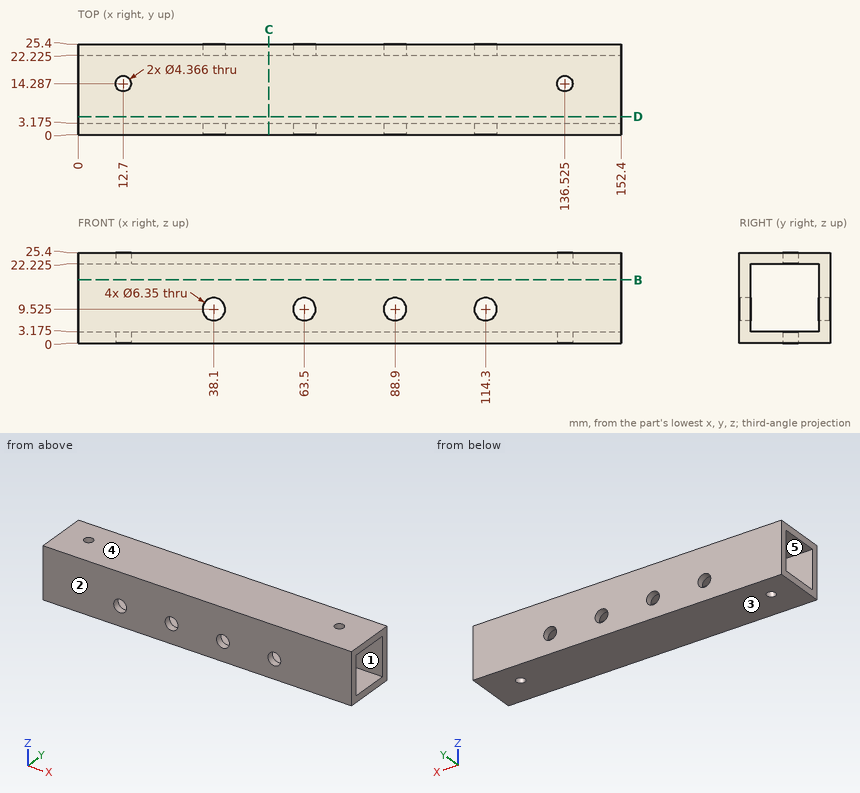
Can you work these out from the drawing? Everything is in mm from the part's minimum corner. A direction names the side the tool comes from. Round coordinates to 2 decimals unless told otherwise and drop trailing zeros. Loops run counter-clockwise (first coordinate to the right, second up) from the corner with the lowest first, then second, coordinate; pieces in that order, holes last. Notation, with made-up numbers: M 85.5,21.5 L 127.5,21.5 A26 cw 127.5,58.5 Z; hole C -11,-14 d1. An arc over 180 degrees is marked long. Answer in a Markdown table with one row per item.
1. If we section it at C-C, the plane x = 53.5: Please give me the cut outline in (y, z) (1 decimal).
Established:
| item | result |
|---|---|
| outline | M 0,0 L 25.4,0 L 25.4,25.4 L 0,25.4 Z; hole M 3.2,3.2 L 22.2,3.2 L 22.2,22.2 L 3.2,22.2 Z |
2. On a 3-axis mill with a long thin cutter (end or side, diameter ignored), from which of +Z, -Z, +X, -X, +Y, -Y can I reach the whole of each face in a straight line? I mean the marked faces 4 and 5. Say none if no direction works.
Established:
| item | result |
|---|---|
| face 4 | +Z, +X, -X, +Y, -Y |
| face 5 | +X, -X |
3. Thinking about a two-plate mould opening in Y: for the marked faces 1, 2 and 3, which applies, pulls with the +Y half, pulls with the -Y half, needs draft (parallel to the pull), parting line crosses it, or undercut?
Established:
| item | result |
|---|---|
| face 1 | undercut |
| face 2 | pulls with the -Y half |
| face 3 | needs draft |
4. Please list where these lines run through material, in increasing order: line 1 (Y direction, x = 12.7, z = 22.95) (1 decimal); line 2 (Y direction, x = 86.5, z = 4.5) (1 decimal). Write a range as from..to.
Established:
| item | result |
|---|---|
| line 1 | 0..12.1, 16.5..25.4 |
| line 2 | 0..3.2, 22.2..25.4 |
5. If we section it at B-B, the plane z = 17.75: Please give me the cut outline in (x, y) (1 decimal).
Established:
| item | result |
|---|---|
| outline | M 0,0 L 152.4,0 L 152.4,3.2 L 0,3.2 Z; M 0,22.2 L 152.4,22.2 L 152.4,25.4 L 0,25.4 Z |
